```python
from build123d import *

# Parameters (mm, degrees)
CROQUIS2_R              = 2
SALIENTE_EXTRUIR2_DEPTH = 3


with BuildPart() as part:
    # Croquis2 → Saliente-Extruir2 (new body)
    with BuildSketch(Plane.XY):
        with BuildLine():
            Line((0, 0), (0, 80))
            Line((0, 80), (0, 235.988905846))
            ThreePointArc((0, 235.988905846), (16.416079704, 275.620828109), (56.048001966, 292.036907812))
            Line((56.048001966, 292.036907812), (189.951998034, 292.036907812))
            ThreePointArc((189.951998034, 292.036907812), (229.583920296, 275.620828109), (246, 235.988905846))
            Line((246, 235.988905846), (246, 180))
            Line((246, 180), (246, -30))
            Line((246, -30), (140, -30))
            Line((140, -30), (110, -30))
            Line((110, -30), (30, -30))
            ThreePointArc((30, -30), (8.786796564, -21.213203436), (0, 0))
        make_face()
        with Locations((20, -10)):
            Circle(CROQUIS2_R, mode=Mode.SUBTRACT)
        with Locations(Location((120, -10, 0), (0, 0, 180))):
            Circle(CROQUIS2_R, mode=Mode.SUBTRACT)
        with Locations((120, 90)):
            Circle(CROQUIS2_R, mode=Mode.SUBTRACT)
        with Locations(Location((20, 90, 0), (0, 0, 180))):
            Circle(CROQUIS2_R, mode=Mode.SUBTRACT)
        with Locations((150, 170)):
            Circle(CROQUIS2_R, mode=Mode.SUBTRACT)
        with Locations(Location((236, 170, 0), (0, 0, 180))):
            Circle(CROQUIS2_R, mode=Mode.SUBTRACT)
        with Locations((236, -20)):
            Circle(CROQUIS2_R, mode=Mode.SUBTRACT)
        with Locations(Location((150, -20, 0), (0, 0, 180))):
            Circle(CROQUIS2_R, mode=Mode.SUBTRACT)
    extrude(amount=SALIENTE_EXTRUIR2_DEPTH)


solid = part.part
```
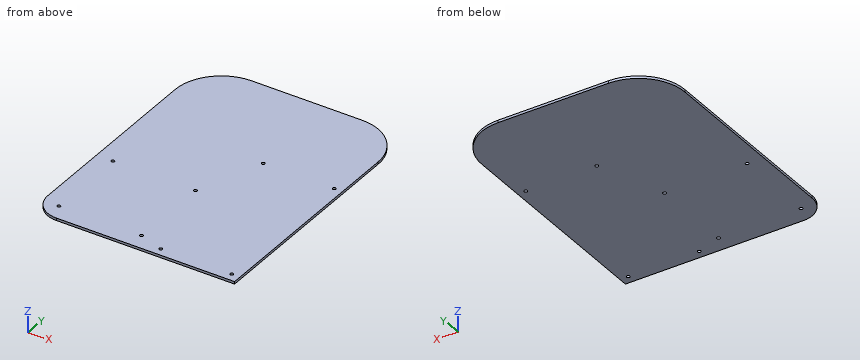
Design review of the part built by this model. Coordinates are the model's own, in mm. Round coordinates to 2 decimals unless told otherwise and drop trailing zeros. Order: outer loops, then holes, each group sorted by start corner. A loop starts at its lowest first (then second) coordinate and runs counter-clockwise, first axis right, second up. Notation, with made-up numbers: (85.5, 6.25) - (98.5, 6.25) arc R29 ccw to (98.5, 41.25) - close; hole circle Ø10 at (-25.5, 40). An arc over 180 degrees is marked (long way). One line per question, with ' | ' between items.
Item 1: Take a section at A-A, the plane x = 219. Write out the cut boundary in (y, z).
Checks:
outline: (-30, 0) - (283.92, 0) - (283.92, 3) - (-30, 3) - close
Item 2: Wall thickness on line 1 (X direction, y = 170, z = 1.9); line 2 (Y direction, x = 150, z = 2.45); line 3 (Y direction, x = 236, z = 1.5): over which ranges is each line inside the solid? List them lowest first. Write a range as [from, to].
Checks:
line 1: [0, 148], [152, 234], [238, 246] | line 2: [-30, -22], [-18, 168], [172, 292.04] | line 3: [-30, -22], [-18, 168], [172, 267.94]
Item 3: For P1, Ø3.5, axis at x = 150, y = 170, coming from the +Z side; P2, Ø6.5, axis at x = 150, y = -20, coming from the -Z side, all flat-tipped, find the tip position at first contact; note any pin that passes through.
Checks:
P1: through | P2: z = 0
